Verification items for the finished model (mm, model axes). A direction names the side the tool comes from. Coordinates: 2 decimals unless noted, no trailing zeros. Loops run counter-clockwise (first coordinate to the right, second up) from the corner with the lowest first, then second, coordinate; pieces in that order, holes last. Notation, with made-up numbers: (20, 87) - (48, 87) arc R23 cw to (48, 96) - close; hole circle Ø4 at (47.5, 24.25). An arc over 180 degrees is marked (long way). Answer as CSV lines item,"result". Start each with the question number.
1. Release check for a two-part mould opening along Z. For faces 1 (the flat face through (8, 9.6, -4)), 2 (the cylindrical face through (3.28, 10.39, -6.29)), 3 (the cylindrical face through (11.207, 8.789, -3.896)), 4 (the flat face through (7.89, 4.73, -12.06)) record: pulls with the +Z half, pulls with the -Z half, needs draft (parallel to the pull), parting line crosses it, or undercut.
2. Gauge pin test, flat ends, axial feed: P1, Ø1.8, axis at x = 11.5, z = -4, coming from the -Y side; P2, Ø4, axis at x = 4.5, y = 8.5, coming from the +Z side; P3, Ø1.4, axis at x = 4, z = -4, coming from the -Y side. Record the tip position at first contact, or that the pin passes through.
3. Set-up check for faces 5 (the flat face through (1.6, 3, -6)), 6 (the cylindrical face through (9.976, 10.389, -5.29)), 7 (the flat face through (4, 11.2, -4)): record each of +Z, -Z, +X, -X, +Y, -Y from which the full face is reachable in a straight line by a thin tool's end or side.
4. Material ranges on line 1 (X direction, y = 8.5, z = -4); line 2 (X direction, y = 3, z = -5.75); line 3 (Z direction, x = 7.75, y = 3.25), recorded low to high. Write a range as [from, to].
5. Cross-section at B-B (x = 12). Enter the section's corners in (y, z).
6. Cross-section at D-D (y = 8.5). Enter the section's corners in (x, z), plus the area to 3 significant figures.
7. Cross-section at A-A (z = -4). Enter the section's corners in (x, y).
8. Cross-section at C-C (y = 4.75). Enter the section's corners in (x, z), plus the area to 3 significant figures.
```python
from build123d import *

# Parameters (mm, degrees)
BOSS_EXTRUDE1_DEPTH = 16
SKETCH2_R           = 2.4
BOSS_EXTRUDE2_DEPTH = 1.6
LPATTERN1_COUNT     = 2
LPATTERN1_PITCH     = 8
SHELL1_T            = -1.6


with BuildPart() as part:
    # Sketch1 → Boss-Extrude1 (new body)
    with BuildSketch(Plane(origin=(0, 0, 0), x_dir=(0, 0, -1), z_dir=(1, 0, 0))):
        Polygon((0, 0), (16, 0), (8, 9.6), (0, 9.6), align=None)
    extrude(amount=BOSS_EXTRUDE1_DEPTH)

    # Sketch2 → Boss-Extrude2 (add)
    with BuildSketch(Plane(origin=(0, 9.6, 0), x_dir=(1, 0, 0), z_dir=(0, 1, 0))):
        with Locations(Location((4, 4, 0), (0, 0, 90))):
            Circle(SKETCH2_R)
    boss_extrude2 = extrude(amount=BOSS_EXTRUDE2_DEPTH)

    # LPattern1: Boss-Extrude2 ×2
    with Locations(*[(i * LPATTERN1_PITCH, 0, 0) for i in range(1, LPATTERN1_COUNT)]):
        add(boss_extrude2)

    # Shell1
    shell1_openings = [part.faces().sort_by_distance(p)[0] for p in [
        (8, 0, -8),
    ]]
    offset(amount=SHELL1_T, openings=shell1_openings, kind=Kind.INTERSECTION)


solid = part.part
```
Values follow:
1,face 1,"needs draft"
1,face 2,"parting line crosses it"
1,face 3,"undercut"
1,face 4,"pulls with the -Z half"
2,P1,"stops at y = 8"
2,P2,"stops at z = 0"
2,P3,"stops at y = 9.6"
3,face 5,"-Y"
3,face 6,"+Y"
3,face 7,"+Z, -Z, +X, -X, +Y"
4,line 1,"x = [0, 3.2], [4.8, 11.2], [12.8, 16]"
4,line 2,"x = [0, 1.6], [14.4, 16]"
4,line 3,"z = [-13.29, -11.21], [-1.6, 0]"
5,outline,"(0, -16) - (9.6, -8) - (9.6, -6.4) - (11.2, -6.4) - (11.2, -1.6) - (9.6, -1.6) - (9.6, 0) - (0, 0) - (0, -1.6) - (8, -1.6) - (8, -3.2) - (9.6, -3.2) - (9.6, -4.8) - (8, -4.8) - (8, -7.25) - (0, -13.92) - close"
6,outline,"(0, -8.92) - (16, -8.92) - (16, 0) - (0, 0) - close; hole circle Ø1.6 at (4, -4); hole circle Ø1.6 at (12, -4)"
6,area,"139 mm²"
7,outline,"(0, 0) - (1.6, 0) - (1.6, 8) - (3.2, 8) - (3.2, 9.6) - (4.8, 9.6) - (4.8, 8) - (11.2, 8) - (11.2, 9.6) - (12.8, 9.6) - (12.8, 8) - (14.4, 8) - (14.4, 0) - (16, 0) - (16, 9.6) - (14.4, 9.6) - (14.4, 11.2) - (9.6, 11.2) - (9.6, 9.6) - (6.4, 9.6) - (6.4, 11.2) - (1.6, 11.2) - (1.6, 9.6) - (0, 9.6) - close"
8,outline,"(0, -12.04) - (16, -12.04) - (16, 0) - (0, 0) - close; hole (1.6, -9.96) - (14.4, -9.96) - (14.4, -1.6) - (1.6, -1.6) - close"
8,area,"85.7 mm²"
